Input: part model. Units: mm. Frame: model coordinates. A direction names the side the tool comes from. Round coordinates to 2 decimals unless told otherwise and drop trailing zeros. Loops run counter-clockwise (first coordinate to the right, second up) from the corner with the lowest first, then second, coordinate; pieces in that order, holes last. Notation, with made-up numbers: (-9, 6) -> (38, 6) arc R14 cw to (38, 33) -> close; hole circle Ø11 at (-24, -23.5). An arc over 180 degrees is marked (long way). One line per question, with ' | ' between items. Start each with the question number.
Q1. Cut plane C-C on x = -77.5. Return loops of the section in (y, z), and give its area (3 significant figures).
Q2. Material intervals for L1, parallel to Z at x = -70, y = -18.3; L2, parallel to Z at x = -100.5, y = -10; L3, parallel to X at y = -4.5, z = 120.5, sorted ascending.
Q3. Cut plane D-D on x = -39. Return loops of the section in (y, z).
Q4. Contact query for flat-ended pins moving along their axis: P1, Ø1.5, axis at x = -50, z = 108.5, coming from the +Y side; P2, Ø11, axis at x = -69.5, z = 125.5, coming from the -Y side; P3, Ø1.5, axis at y = -11.5, z = 63, coming from the +X side; P4, Ø8, axis at y = -16, z = 108.5, coming from the +X side. Output: stop coordinate, or through.
Q5. Cut plane A-A on y = -17. Return loops of the section in (x, z), and give its area (3 significant figures).
Q6. Access query for faces 1 (the face through (-70, -15, 122)), 2 (the face through (-22.2, -9.9, 71.8)). Directions: +Z, -Z, +X, -X, +Y, -Y. A direction counts if a zero-diameter tool reaches every point of the face in a straight line with its end or side. Return the directions, or none.
Q7. Cut plane B-B on y = -2.5. Return loops of the section in (x, z), and give its area (3 significant figures).
from build123d import *

# Parameters (mm, degrees)
F0_W     = 140
F0_H     = 20
F1_DEPTH = 20
F3_DEPTH = 5


with BuildPart() as f1:
    # F0 (on Front) → F1 (new body)
    with BuildSketch(Plane.XZ):
        with BuildLine():
            ThreePointArc((-60.8786071337, 140), (-70, 141.578780142), (-79.1213928663, 140))
            Line((-79.1213928663, 140), (-60.8786071337, 140))
        make_face()
        with Locations((-70, 10)):
            Rectangle(F0_W, F0_H)
        with BuildLine():
            Line((-60.8786071337, 140), (-79.1213928663, 140))
            ThreePointArc((-79.1213928663, 140), (-88.6364525268, 134.16805413), (-95, 125))
            ThreePointArc((-95, 125), (-75.3872103911, 87.8412774691), (-42.8612134521, 114.439993594))
            ThreePointArc((-42.8612134521, 114.439993594), (-43.401283875, 119.8272039851), (-45, 125))
            ThreePointArc((-45, 125), (-51.3635474732, 134.16805413), (-60.8786071337, 140))
        make_face()
        with BuildLine():
            Line((-95, 125), (-140, 20))
            Line((-140, 20), (0, 20))
            Line((0, 20), (-45, 125))
            ThreePointArc((-45, 125), (-43.401283875, 119.8272039851), (-42.8612134521, 114.439993594))
            ThreePointArc((-42.8612134521, 114.439993594), (-75.3872103911, 87.8412774691), (-95, 125))
        make_face()
    extrude(amount=F1_DEPTH)

    # F2 (on face) → F3 (cut)
    with BuildSketch(Plane.XZ.offset(20)):
        with BuildLine():
            ThreePointArc((-70, 132.578780142), (-77.7781745931, 113.8006055489), (-59, 121.578780142))
            ThreePointArc((-59, 121.578780142), (-62.2218254069, 129.356954735), (-70, 132.578780142))
        make_face()
    extrude(amount=-F3_DEPTH, mode=Mode.SUBTRACT)


solid = f1.part
Results:
1) outline: (-20, 0) -> (0, 0) -> (0, 140.52) -> (-20, 140.52) -> (-20, 129.63) -> (-15, 129.63) -> (-15, 113.53) -> (-20, 113.53) -> close | area: 2,730 mm^2
2) L1: 0 to 110.58, 132.58 to 141.58 | L2: 0 to 112.17 | L3: -96.93 to -43.07
3) outline: (-20, 0) -> (0, 0) -> (0, 111) -> (-20, 111) -> close
4) P1: y = 0 | P2: y = -15 | P3: x = -18.11 | P4: x = -36.21
5) outline: (-140, 0) -> (0, 0) -> (0, 20) -> (-45, 125) arc R27.14 ccw to (-95, 125) -> (-140, 20) -> close; hole circle Ø22 at (-70, 121.58) | area: 13,000 mm^2
6) face 1: -Y | face 2: +Z, +X, +Y, -Y
7) outline: (-140, 0) -> (0, 0) -> (0, 20) -> (-45, 125) arc R27.14 ccw to (-95, 125) -> (-140, 20) -> close | area: 13,400 mm^2
